CAD build for the part. Positions are in the model's coordinates, mm. A direction names the side the tool comes from. Round coordinates to 2 decimals unless told otherwise and drop trailing zeros. Order: outer loops, then holes, each group sorted by start corner. A loop starts at its lowest first (then second) coordinate and runs counter-clockwise, first axis right, second up.
```python
from build123d import *

# Parameters (mm, degrees)
BOSS_EXTRUDE1_DEPTH = 60
FILLET1_R           = 1
SKETCH2_R           = 3
CUT_EXTRUDE1_DEPTH  = 2


with BuildPart() as part:
    # Sketch1 → Boss-Extrude1 (new body)
    with BuildSketch(Plane.XY):
        Polygon((-15, 0), (-15, 2), (-28, 2), (-28, 28), (28, 28), (28, 2), (15, 2), (15, 0), (30, 0), (30, 30), (-30, 30), (-30, 0), align=None)
    extrude(amount=BOSS_EXTRUDE1_DEPTH)

    # Fillet1
    fillet1_edges = [part.edges().sort_by_distance(p)[0] for p in [
        (28, 2, 30),
        (28, 28, 30),
        (-28, 28, 30),
        (-28, 2, 30),
        (-30, 0, 30),
        (-30, 30, 30),
        (30, 30, 30),
        (30, 0, 30),
    ]]
    fillet(fillet1_edges, radius=FILLET1_R)

    # Sketch2 → Cut-Extrude1 (cut)
    with BuildSketch(Plane(origin=(0, 30, 0), x_dir=(1, 0, 0), z_dir=(0, 1, 0))):
        with Locations(Location((0, -30, 0), (0, 0, 180))):
            Circle(SKETCH2_R)
    extrude(amount=-CUT_EXTRUDE1_DEPTH, mode=Mode.SUBTRACT)


solid = part.part
```
1. Pin check, flat tips, straight feed: P1, Ø9.5, axis at x = 0, z = 30, coming from the -Y side; P2, Ø16, axis at x = 11, z = 25.5, coming from the -Y side. Stop position of each tip, or through.
2. Drill centre lines: line 1 (Y direction, x = 24, z = 48); line 2 (X direction, y = 4, z = 28); line 3 (Z direction, x = 0, y = 29.25). Where is each one in solid material? Low to high.
3. Cut at A-A, the plane y = 22. Write the cut outline in (x, z).
4. Tool access for faces 1 (the face through (-15, 1, 30)), 2 (the face through (-6, 28, 30)), 3 (the face through (-2.4, 28.4, 0)): list every direction of +Z, -Z, +X, -X, +Y, -Y with a clear straight run to the whole face (end or side of a thin tool).
5. Cut at D-D, the plane z = 18. Write the cut outline in (x, y).
6. Cut at B-B, the plane x = 23. Write the cut outline in (y, z), and give its area (3 significant figures).
7. Mould opens along Y. For faces 4 (the face through (22, 0, 30)), 5 (the face through (-30, 15, 30)), 6 (the face through (-28, 15, 30)) say: released by +Y, released by -Y, zero draft, split by the parting line, or undercut.
8. Cut at C-C, the plane z = 30. Write the cut outline in (x, y).
Outcome:
1. P1: stops at y = 28
1. P2: stops at y = 0
2. line 1: y = 0 to 2, 28 to 30
2. line 2: x = -30 to -28, 28 to 30
2. line 3: z = 0 to 27, 33 to 60
3. outline: (-30, 0) - (-28, 0) - (-28, 60) - (-30, 60) - close; (28, 0) - (30, 0) - (30, 60) - (28, 60) - close
4. face 1: +Z, -Z, -Y
4. face 2: +Z, -Z
4. face 3: -Z, +X, -X, +Y, -Y
5. outline: (-30, 1) arc R1 ccw to (-29, 0) - (-15, 0) - (-15, 2) - (-27, 2) arc R1 cw to (-28, 3) - (-28, 27) arc R1 cw to (-27, 28) - (27, 28) arc R1 cw to (28, 27) - (28, 3) arc R1 cw to (27, 2) - (15, 2) - (15, 0) - (29, 0) arc R1 ccw to (30, 1) - (30, 29) arc R1 ccw to (29, 30) - (-29, 30) arc R1 ccw to (-30, 29) - close
6. outline: (0, 0) - (2, 0) - (2, 60) - (0, 60) - close; (28, 0) - (30, 0) - (30, 60) - (28, 60) - close
6. area: 240 mm2
7. face 4: released by -Y
7. face 5: zero draft
7. face 6: undercut
8. outline: (-30, 1) arc R1 ccw to (-29, 0) - (-15, 0) - (-15, 2) - (-27, 2) arc R1 cw to (-28, 3) - (-28, 27) arc R1 cw to (-27, 28) - (-3, 28) - (-3, 30) - (-29, 30) arc R1 ccw to (-30, 29) - close; (3, 28) - (27, 28) arc R1 cw to (28, 27) - (28, 3) arc R1 cw to (27, 2) - (15, 2) - (15, 0) - (29, 0) arc R1 ccw to (30, 1) - (30, 29) arc R1 ccw to (29, 30) - (3, 30) - close
